Geometry: final body of the model. Coordinates: model frame, mm. Give positions to 0.01 mm unless a question says otherwise; leave off trailing zeros. Write each loop counter-clockwise with the first axis right and the second up, starting at its lowest first coordinate (ties: lowest second). Pieces come first, ordered by that corner, then holes. Notation, with made-up numbers: (67.25, -20.5) - (103.25, -20.5) arc R26 cw to (103.25, -6.5) - close; hole circle Ø7 at (10, -27.5). An arc over 180 degrees is marked (long way). Return JSON: item names as keys, results as strings.
from build123d import *

# Parameters (mm, degrees)
F2_DEPTH = 11.90625


# Not quite as in the source:
# - a variable given as a bare number and used for a length is read in inches; the dataset says mm whatever the document's units were


with BuildPart() as f2:
    # F1 (on Front) → F2 (new body)
    with BuildSketch(Plane.XZ):
        with BuildLine():
            Line((914.4, 406.4), (0, 406.4))
            Line((0, 406.4), (0, 203.2))
            Line((0, 203.2), (117.3175746993, 0))
            Line((117.3175746993, 0), (222.25, 0))
            Line((222.25, 0), (222.25, 203.2))
            ThreePointArc((222.25, 203.2), (228.6, 209.55), (234.95, 203.2))
            Line((234.95, 203.2), (234.95, 0))
            Line((234.95, 0), (679.45, 0))
            Line((679.45, 0), (679.45, 203.2))
            ThreePointArc((679.45, 203.2), (685.8, 209.55), (692.15, 203.2))
            Line((692.15, 203.2), (692.15, 0))
            Line((692.15, 0), (797.0824253007, 0))
            Line((797.0824253007, 0), (914.4, 203.2))
            Line((914.4, 203.2), (1031.7175746993, 0))
            Line((1031.7175746993, 0), (1136.65, 0))
            Line((1136.65, 0), (1136.65, 203.2))
            ThreePointArc((1136.65, 203.2), (1143, 209.55), (1149.35, 203.2))
            Line((1149.35, 203.2), (1149.35, 0))
            Line((1149.35, 0), (1593.85, 0))
            Line((1593.85, 0), (1593.85, 203.2))
            ThreePointArc((1593.85, 203.2), (1600.2, 209.55), (1606.55, 203.2))
            Line((1606.55, 203.2), (1606.55, 0))
            Line((1606.55, 0), (1711.4824253007, 0))
            Line((1711.4824253007, 0), (1828.8, 203.2))
            Line((1828.8, 203.2), (1828.8, 406.4))
            Line((1828.8, 406.4), (914.4, 406.4))
        make_face()
        with BuildLine():
            Line((393.7, 368.3), (457.2, 368.3))
            Line((457.2, 368.3), (520.7, 368.3))
            ThreePointArc((520.7, 368.3), (539.75, 349.25), (520.7, 330.2))
            Line((520.7, 330.2), (457.2, 330.2))
            Line((457.2, 330.2), (393.7, 330.2))
            ThreePointArc((393.7, 330.2), (374.65, 349.25), (393.7, 368.3))
        make_face(mode=Mode.SUBTRACT)
        with BuildLine():
            Line((1308.1, 368.3), (1371.6, 368.3))
            Line((1371.6, 368.3), (1435.1, 368.3))
            ThreePointArc((1435.1, 368.3), (1454.15, 349.25), (1435.1, 330.2))
            Line((1435.1, 330.2), (1371.6, 330.2))
            Line((1371.6, 330.2), (1308.1, 330.2))
            ThreePointArc((1308.1, 330.2), (1289.05, 349.25), (1308.1, 368.3))
        make_face(mode=Mode.SUBTRACT)
    extrude(amount=F2_DEPTH)


solid = f2.part
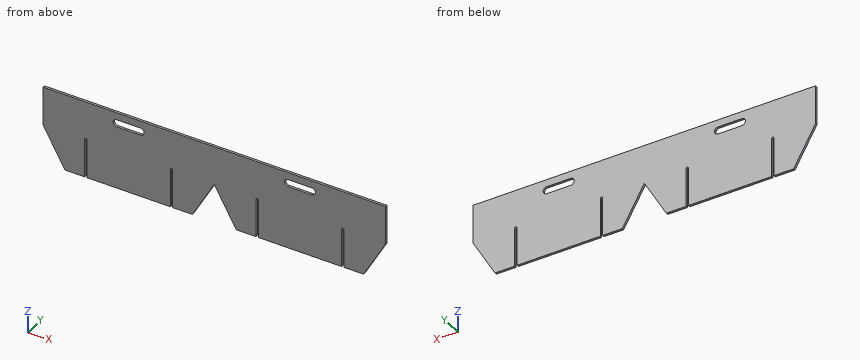
Q1. Section query B-B, the plane y = -2.75. Count the separate pieces of the cut face and the enclosed holes in it, plus the area to 3 significant figures.
Answer key:
{"separate pieces": "1", "enclosed holes": "2", "area": "673,000 mm^2"}
Q2. Material intervals for probe 1 along Z at (x, y) = (1375.5, -9); probe 2 along X at (y, z) = (-1.5, 140.5); probe 3 along X at (y, z) = (-3.5, 200), sorted ascending. Write a range as [from, to].
Answer key:
{"probe 1": "z = [0, 330.2], [368.3, 406.4]", "probe 2": "x = [36.2, 222.25], [234.95, 679.45], [692.15, 878.2], [950.6, 1136.65], [1149.35, 1593.85], [1606.55, 1792.6]", "probe 3": "x = [1.85, 222.25], [234.95, 679.45], [692.15, 912.55], [916.25, 1136.65], [1149.35, 1593.85], [1606.55, 1826.95]"}
Q3. Section query A-A, the plane z = 349.25. Return the cut outline in (x, y), plus the area to 3 significant figures.
Answer key:
{"outline": "(0, -11.91) - (374.65, -11.91) - (374.65, 0) - (0, 0) - close; (539.75, -11.91) - (1289.05, -11.91) - (1289.05, 0) - (539.75, 0) - close; (1454.15, -11.91) - (1828.8, -11.91) - (1828.8, 0) - (1454.15, 0) - close", "area": "17,800 mm^2"}
Q4. Section query C-C, the plane z = 45. Return the cut outline in (x, y), plus the area to 3 significant figures.
Answer key:
{"outline": "(91.34, -11.91) - (222.25, -11.91) - (222.25, 0) - (91.34, 0) - close; (234.95, -11.91) - (679.45, -11.91) - (679.45, 0) - (234.95, 0) - close; (692.15, -11.91) - (823.06, -11.91) - (823.06, 0) - (692.15, 0) - close; (1005.74, -11.91) - (1136.65, -11.91) - (1136.65, 0) - (1005.74, 0) - close; (1149.35, -11.91) - (1593.85, -11.91) - (1593.85, 0) - (1149.35, 0) - close; (1606.55, -11.91) - (1737.46, -11.91) - (1737.46, 0) - (1606.55, 0) - close", "area": "16,800 mm^2"}
Q5. Pin query (flat end, axial travel): P1, Ø6, axis at y = -7.5, z = 92, coming from the +X side; P2, Ø3.5, axis at y = -6.5, z = 54, coming from the -X side; P3, Ø6, axis at y = -4.5, z = 62, coming from the +X side. Return the tip coordinate at first contact, or that it passes through.
Answer key:
{"P1": "stops at x = 1766.33", "P2": "stops at x = 85.13", "P3": "stops at x = 1749.01"}
